Geometry check sheet. Reference: the model listing, model coordinates, mm. Face numbers are marked on the shaded views. A direction names the side the tool comes from. Round coordinates to 2 decimals unless told otherwise and drop trailing zeros. Order: outer loops, then holes, each group sorted by start corner. A loop starts at its lowest first (then second) coordinate and runs counter-clockwise, first axis right, second up.
(1) Sectioned sample at C-C (x = 1). Record the boundary of the cut face in (y, z).
(2) Sectioned sample at D-D (z = 7.5). Record the boundary of the cut face in (x, y).
(3) Go/stop test with flat-tipped pins: pin 1 (1 mm diameter, centred on x = 11.5, y = -6.5, fed in from -Z); pin 2 (1.6 mm diameter, centred on x = -1.5, y = 18, fed in from +Z); pin 3 (4 mm diameter, centred on x = -15, y = 9.5, fed in from +Z); pin 4 (0.8 mm diameter, centred on y = 18.5, z = 2, fed in from -X). Record where each tip stops, or that it passes through.
(4) Set-up check for the marked faces 1, 2, 3 and 4: record each of +Z, -Z, +X, -X, +Y, -Y from which the full face is reachable in a straight line by a thin tool's end or side.
(5) Sectioned sample at A-A (z = 2.25). Record the boundary of the cut face in (x, y).
(6) Sectioned sample at B-B (y = -5.5). Record the boundary of the cut face in (x, z), plus the area to 3 significant figures.
(7) Material ranges on line 1 along Z through (x, y) = (-13.5, -16.5); line 2 along X through (y, z) = (-4, 9.5); line 3 along Y through (x, z) = (4.5, 5.25), recorded low to high.
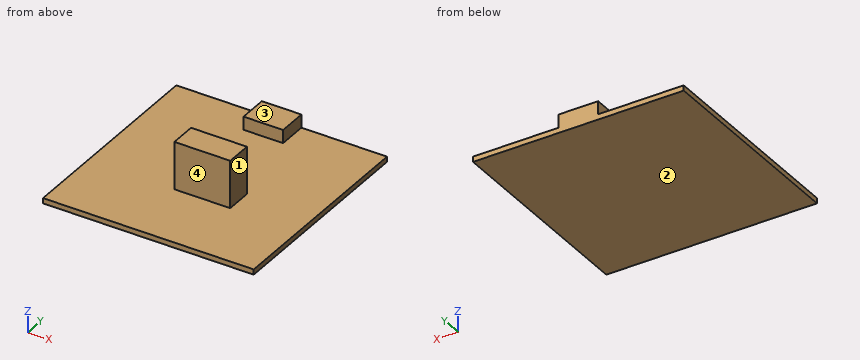
from build123d import *

# Parameters (mm, degrees)
F0_W     = 40
F0_H     = 40
F1_DEPTH = 1
F2_W     = 10.6
F2_H     = 5
F3_DEPTH = 9
F2_W_2   = 7.5
F2_H_2   = 5.5
F4_DEPTH = 2.5


with BuildPart() as f1:
    # F0 (on Top) → F1 (new body)
    with BuildSketch(Plane.XY):
        Rectangle(F0_W, F0_H)
    extrude(amount=F1_DEPTH)

    # F2 (on face) → F3 (join)
    with BuildSketch(Plane.XY.offset(1)):
        with Locations((1.7, -4)):
            Rectangle(F2_W, F2_H)
    extrude(amount=F3_DEPTH)

    # F2 (on face) → F4 (join)
    with BuildSketch(Plane.XY.offset(1)):
        with Locations((0, 17.25)):
            Rectangle(F2_W_2, F2_H_2)
    extrude(amount=F4_DEPTH)


solid = f1.part
Answer below:
1. outline: (-20, 0) - (20, 0) - (20, 3.5) - (14.5, 3.5) - (14.5, 1) - (-1.5, 1) - (-1.5, 10) - (-6.5, 10) - (-6.5, 1) - (-20, 1) - close
2. outline: (-3.6, -6.5) - (7, -6.5) - (7, -1.5) - (-3.6, -1.5) - close
3. pin 1: stops at z = 0
3. pin 2: stops at z = 3.5
3. pin 3: stops at z = 1
3. pin 4: stops at x = -3.75
4. face 1: +Z, +X, +Y, -Y
4. face 2: -Z, +X, -X, +Y, -Y
4. face 3: +Z, +X, -X, +Y
4. face 4: +Z, +X, -X, -Y
5. outline: (-3.75, 14.5) - (3.75, 14.5) - (3.75, 20) - (-3.75, 20) - close; (-3.6, -6.5) - (7, -6.5) - (7, -1.5) - (-3.6, -1.5) - close
6. outline: (-20, 0) - (20, 0) - (20, 1) - (7, 1) - (7, 10) - (-3.6, 10) - (-3.6, 1) - (-20, 1) - close
6. area: 135 mm2
7. line 1: z = 0 to 1
7. line 2: x = -3.6 to 7
7. line 3: y = -6.5 to -1.5
